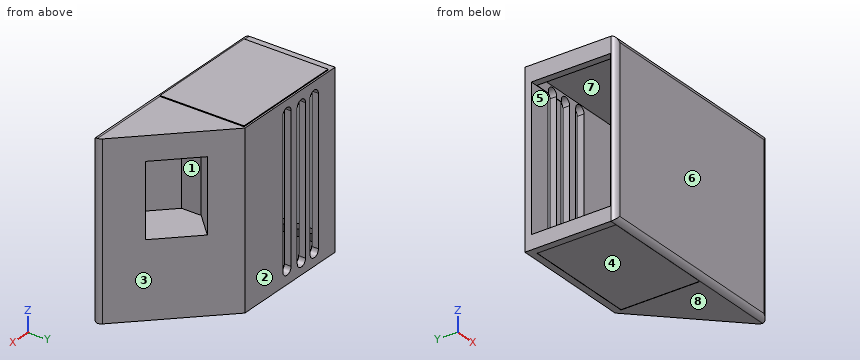
from build123d import *

# Parameters (mm, degrees)
Y_KSEKLIK_EKSTR_ZYON1_DEPTH = 84.582
IZIM2_W                     = 56.613252044
IZIM2_H                     = 38.905458561
KES_EKSTR_ZYON1_DEPTH       = 84.582
IZIM3_W                     = 24.859999106
IZIM3_H                     = 35.80382045
KES_EKSTR_ZYON2_DEPTH       = 22.86
IZIM4_W                     = 56.56840029
IZIM4_H                     = 3.7507773
Y_KSEKLIK_EKSTR_ZYON3_DEPTH = 41.402
IZIM5_W                     = 56.873307594
IZIM5_H                     = 3.441337166
Y_KSEKLIK_EKSTR_ZYON4_DEPTH = 41.402
KES_EKSTR_ZYON3_DEPTH       = 20.828
IZIM7_W                     = 69.770370065
IZIM7_H                     = 38.93587287
KES_EKSTR_ZYON4_DEPTH       = 20.828
RADYUS1_R                   = 2.54


with BuildPart() as part:
    # Çizim1 → Yükseklik-Ekstrüzyon1 (new body)
    with BuildSketch(Plane.XY):
        Polygon((-100.117298217, 48.908980301), (-39.325061833, 48.908980301), (5.581137472, 4.002780997), (-100.117298217, 4.002780997), align=None)
    extrude(amount=Y_KSEKLIK_EKSTR_ZYON1_DEPTH)

    # Çizim2 → Kes-Ekstrüzyon1 (cut)
    with BuildSketch(Plane.XY.offset(84.582)):
        with Locations((-68.275200444, 26.094986488)):
            Rectangle(IZIM2_W, IZIM2_H)
    extrude(amount=-KES_EKSTR_ZYON1_DEPTH, mode=Mode.SUBTRACT)

    # Çizim3 → Kes-Ekstrüzyon2 (cut)
    with BuildSketch(Plane(origin=(4.791959234, 4.791959234, 0), x_dir=(0.7071067811865521, -0.7071067811865429, 0), z_dir=(0.7071067811865429, 0.7071067811865521, 0))):
        with Locations((-34.88056776, -54.904893427)):
            Rectangle(IZIM3_W, IZIM3_H)
    extrude(amount=-KES_EKSTR_ZYON2_DEPTH, mode=Mode.SUBTRACT)

    # Çizim4 → Yükseklik-Ekstrüzyon3 (add)
    with BuildSketch(Plane(origin=(0, 6.642257207, 0.5213718), x_dir=(1, 0, 0), z_dir=(0, 1, 0))):
        with Locations((-68.26547223, -82.621441536)):
            Rectangle(IZIM4_W, IZIM4_H)
    extrude(amount=Y_KSEKLIK_EKSTR_ZYON3_DEPTH)

    # Çizim5 → Yükseklik-Ekstrüzyon4 (add)
    with BuildSketch(Plane(origin=(0, 6.642257207, 0), x_dir=(1, 0, 0), z_dir=(0, 1, 0))):
        with Locations((-68.314463999, -1.839596634)):
            Rectangle(IZIM5_W, IZIM5_H)
    extrude(amount=Y_KSEKLIK_EKSTR_ZYON4_DEPTH)

    # Çizim6 → Kes-Ekstrüzyon3 (cut)
    with BuildSketch(Plane(origin=(0, 48.908980301, 0), x_dir=(1, 0, 0), z_dir=(0, 1, 0))):
        with BuildLine():
            Line((-88.870816985, -77.80498522), (-88.870816985, -6.700388759))
            ThreePointArc((-88.870816985, -6.700388759), (-86.078686723, -3.908258497), (-83.286556461, -6.700388759))
            Line((-83.286556461, -6.700388759), (-83.286556461, -77.80498522))
            ThreePointArc((-83.286556461, -77.80498522), (-86.078686723, -80.597115482), (-88.870816985, -77.80498522))
        make_face()
        with BuildLine():
            Line((-80.201988502, -77.524018239), (-80.201988502, -6.419421778))
            ThreePointArc((-80.201988502, -6.419421778), (-77.40985824, -3.627291516), (-74.617727978, -6.419421778))
            Line((-74.617727978, -6.419421778), (-74.617727978, -77.524018239))
            ThreePointArc((-74.617727978, -77.524018239), (-77.40985824, -80.316148501), (-80.201988502, -77.524018239))
        make_face()
        with BuildLine():
            Line((-70.501383696, -78.211655362), (-70.501383696, -7.107058901))
            ThreePointArc((-70.501383696, -7.107058901), (-67.709253434, -4.314928639), (-64.917123172, -7.107058901))
            Line((-64.917123172, -7.107058901), (-64.917123172, -78.211655362))
            ThreePointArc((-64.917123172, -78.211655362), (-67.709253434, -81.003785624), (-70.501383696, -78.211655362))
        make_face()
    extrude(amount=-KES_EKSTR_ZYON3_DEPTH, mode=Mode.SUBTRACT)

    # Çizim7 → Kes-Ekstrüzyon4 (cut)
    with BuildSketch(Plane.ZY.offset(100.117298217)):
        with Locations((41.890344752, 26.266043038)):
            Rectangle(IZIM7_W, IZIM7_H)
    extrude(amount=-KES_EKSTR_ZYON4_DEPTH, mode=Mode.SUBTRACT)

    # Radyus1
    radyus1_edges = [part.edges().sort_by_distance(p)[0] for p in [
        (-47.268080373, 4.002780997, 0),
        (-47.268080373, 4.002780997, 84.582),
        (5.581137472, 4.002780997, 42.291),
        (-100.117298217, 4.002780997, 42.291),
    ]]
    fillet(radyus1_edges, radius=RADYUS1_R)


solid = part.part
Could you check a few things on this model? Use its own coordinates, in mm. Face numbers are marked on the shaded views. A direction names the side the tool comes from. Give positions to 0.01 mm unless a question says otherwise; leave off trailing zeros. Write each loop counter-clockwise with the first axis right and the second up, starting at its lowest first coordinate (ties: lowest second). Pieces come first, ordered by that corner, then holes. Notation, with made-up numbers: (37.25, 9) -> (51.25, 9) arc R14 cw to (51.25, 18) -> close; hole circle Ø7 at (-7, -27.5). An arc over 180 degrees is marked (long way). Answer as a JSON object with one key per item and string values.
Q1. Suppose I cut it at A-A on z = 31.5. Write out the boundary of the cut face in (x, y), then the cut area to 3 significant figures.
Taken from the geometry:
{"outline": "(-100.12, 6.54) arc R2.54 ccw to (-97.58, 4) -> (-0.55, 4) arc R2.54 ccw to (1.25, 8.34) -> (-39.33, 48.91) -> (-64.92, 48.91) -> (-64.92, 45.55) -> (-39.97, 45.55) -> (-39.97, 6.64) -> (-96.58, 6.64) -> (-96.58, 6.8) -> (-100.12, 6.8) -> close; (-100.12, 45.73) -> (-88.87, 45.73) -> (-88.87, 48.91) -> (-100.12, 48.91) -> close; (-83.29, 45.73) -> (-80.2, 45.73) -> (-80.2, 48.91) -> (-83.29, 48.91) -> close; (-74.62, 45.55) -> (-70.5, 45.55) -> (-70.5, 48.91) -> (-74.62, 48.91) -> close", "area": "1,330 mm²"}
Q2. Suppose I cut it at C-C on y = 13. Write out the boundary of the cut face in (x, z) (3 decimals), then the cut area to 3 significant figures.
Taken from the geometry:
{"outline": "(-100.117, 0) -> (-96.582, 0) -> (-96.582, 0.119) -> (-39.969, 0.119) -> (-39.969, 0) -> (-3.416, 0) -> (-3.416, 84.582) -> (-39.969, 84.582) -> (-39.969, 3.56) -> (-96.582, 3.56) -> (-96.582, 7.005) -> (-100.117, 7.005) -> close; (-100.117, 76.776) -> (-96.582, 76.776) -> (-96.582, 84.582) -> (-100.117, 84.582) -> close; (-96.55, 81.267) -> (-39.981, 81.267) -> (-39.981, 85.018) -> (-96.55, 85.018) -> close; hole (-35.745, 37.003) -> (-18.75, 37.003) -> (-18.75, 72.807) -> (-35.745, 72.807) -> close", "area": "2,940 mm²"}
Q3. Will these pins go through, and if not, where does the flat tip stop? pin 1 Ø19.5 at (x, y) = (-76.5, 34.5) entering from -Z; pin 2 Ø14.5 at (x, y) = (-28.5, 22) entering from +Z; pin 3 Ø10 at (y, z) = (19.5, 34) entering from +X.
Taken from the geometry:
{"pin 1": "stops at z = 0.12", "pin 2": "stops at z = 84.58", "pin 3": "stops at x = -4.92"}
Q4. Which directions (+Z, -Z, +X, -X, +Y, -Y) give clear straight access to the entire face, cutting with the end or side of a thin tool? Please do the marked faces 4, 5, 6, 7 and 8.
Taken from the geometry:
{"face 4": "-Z", "face 5": "-X", "face 6": "+Z, -Z, +X, -X, -Y", "face 7": "none", "face 8": "-Z, +X, -X, +Y, -Y"}
Q5. Suppose I cut it at B-B on x = -92.5. Write out the boundary of the cut face in (y, z).
Taken from the geometry:
{"outline": "(4, 2.54) arc R2.54 ccw to (6.54, 0) -> (6.64, 0) -> (6.64, 0.12) -> (45.55, 0.12) -> (45.55, 0) -> (48.91, 0) -> (48.91, 84.58) -> (48.04, 84.58) -> (48.04, 85.02) -> (6.64, 85.02) -> (6.64, 84.58) -> (6.54, 84.58) arc R2.54 ccw to (4, 82.04) -> close; hole (6.64, 3.56) -> (45.55, 3.56) -> (45.55, 7.01) -> (45.73, 7.01) -> (45.73, 76.78) -> (45.55, 76.78) -> (45.55, 81.27) -> (6.64, 81.27) -> close"}
Q6. Please list where these lines run through material, in increasing order: L1, parallel to Y at x = -47.5, z = 45; L2, parallel to Z at x = -81.5, y = 29.5; L3, parallel to Y at x = -81.5, z = 11.5.
Taken from the geometry:
{"L1": "y = 4 to 6.64, 45.55 to 48.91", "L2": "z = 0.12 to 3.56, 81.27 to 85.02", "L3": "y = 4 to 6.64, 45.73 to 48.91"}
Q7. Suppose I cut it at D-D on z = 51.5. Count the separate pieces of the cut face and the enclosed holes in it, then the cut area to 3 significant figures.
Taken from the geometry:
{"separate pieces": "5", "enclosed holes": "0", "area": "786 mm²"}
Q8. We'd pull the mould along X, two halves only. Please class the marked faces 1, 2 and 3: released by +X, released by -X, zero draft, split by the parting line, or undercut.
Taken from the geometry:
{"face 1": "undercut", "face 2": "zero draft", "face 3": "released by +X"}
